Input: part model. Units: mm. Frame: model coordinates. Face numbers are marked on the shaded views. A direction names the side the tool comes from. Coordinates: 2 decimals unless noted, no trailing zeros. Loops run counter-clockwise (first coordinate to the right, second up) from the corner with the lowest first, then second, coordinate; pieces in that order, holes last. Notation, with made-up numbers: (-2, -23) -> (11, -23) arc R26 ccw to (11, -1) -> close; hole circle Ø4 at (56.25, -32). An arc over 180 degrees is marked (long way). Put each result on its own line as item: value. Start each with the question number.
1) Set-up query: the marked faces 1 and 2. Return all of +Z, -Z, +X, -X, +Y, -Y with unobstructed straight access to the full face (end or side cutting, diameter ignored); none if empty.
2) Cut plane A-A (x = 3.3). Return the cut outline in (y, z).
3) Cut plane D-D (y = 4.65). State how many separate pieces and enclosed holes the cut face has, plus the area to 3 significant figures.
4) Material intervals for L1, parallel to X at y = 3.35, z = -10; L2, parallel to X at y = 0.65, z = -8.5; L3, parallel to X at y = 1.15, z = -26, sorted ascending.
5) Cut plane B-B (x = 37). Return the cut outline in (y, z), plus the area to 3 significant figures.
6) Cut plane C-C (x = 56). Return the cut outline in (y, z), plus the area to 3 significant figures.
7) Contact query for flat-ended pins moving along their axis: P1, Ø1.5, axis at x = 26.5, y = 1.5, coming from the -Z side; P2, Ø3, axis at x = 16, z = -17.5, coming from the +Y side (3 decimals); P3, Ø3, axis at x = 25, z = -18.5, coming from the +Y side. Output: stop coordinate, or through.
from build123d import *

# Parameters (mm, degrees)
SKETCH_1_W                 = 60
SKETCH_1_H                 = 30
EXTRUDE_1_DEPTH            = 5.5
HOLE_WIZARD_41_D           = 2.9464
HOLE_WIZARD_41_CBORE_D     = 5.588
HOLE_WIZARD_41_CBORE_DEPTH = 2.9972
CUT_EXTRUDE_START          = -5.5
CUT_EXTRUDE_1_OUTLINE_R    = 2.25
CUT_EXTRUDE_1_OUTLINE_R_2  = 2
CUT_EXTRUDE_1_OUTLINE_R_3  = 1
CUT_EXTRUDE_1_DEPTH        = 5.5
CUT_EXTRUDE_START_2        = -3.5
SKETCH_4_3_R               = 5.5
SKETCH_4_3_R_2             = 2.25
CUT_EXTRUDE_2_DEPTH        = 3.5
CUT_EXTRUDE_START_3        = -3.3
CUT_EXTRUDE_3_DEPTH        = 3.3
HOLE_WIZARD_M3_AT_2_COUNT  = 2
HOLE_WIZARD_M3_AT_2_PITCH  = 14.637281168
HOLE_WIZARD_M3_AT_3_COUNT  = 2
HOLE_WIZARD_M3_AT_3_PITCH  = 36.045110625
HOLE_WIZARD_M3_AT_4_COUNT  = 2
HOLE_WIZARD_M3_AT_4_PITCH  = 33
SKETCH_7_R                 = 5
CUT_EXTRUDE_4_DEPTH        = 69.411439102


# Read off the part's stored shape, not the designer's step: the extrude step
with BuildPart() as part:
    # Sketch 1 → Extrude 1 (new body)
    with BuildSketch(Plane(origin=(0, 0, 0), x_dir=(1, 0, 0), z_dir=(0, 1, 0))):
        with Locations((30, 15)):
            Rectangle(SKETCH_1_W, SKETCH_1_H)
    extrude(amount=EXTRUDE_1_DEPTH)

    # Hole Wizard 41 (through all)
    with Locations(Plane(origin=(0, 5.5, 0), x_dir=(-1, 0, 0), z_dir=(0, 1, 0))):
        with Locations((-47.3, -9), (-3.3, -9), (-25.3, -18), (-3.3, -25), (-56.3, -9), (-56.3, -24)):
            CounterBoreHole(HOLE_WIZARD_41_D / 2, HOLE_WIZARD_41_CBORE_D / 2, HOLE_WIZARD_41_CBORE_DEPTH)

    # Cut-Extrude 1 outline → Cut-Extrude 1 (cut)
    with BuildSketch(Plane(origin=(0, 5.5, 0), x_dir=(1, 0, 0), z_dir=(0, 1, 0)).offset(CUT_EXTRUDE_START)):
        with BuildLine():
            Line((57.765087934, 30), (14.834912066, 30))
            ThreePointArc((14.834912066, 30), (36.3, 20.5), (57.765087934, 30))
        make_face()
        with Locations((36, 14.5)):
            Circle(CUT_EXTRUDE_1_OUTLINE_R)
        with Locations((19.3, 19.8)):
            Circle(CUT_EXTRUDE_1_OUTLINE_R_2)
        with Locations((33.1, 7.4)):
            Circle(CUT_EXTRUDE_1_OUTLINE_R_3)
        with Locations((38.9, 7.4)):
            Circle(CUT_EXTRUDE_1_OUTLINE_R_3)
        with Locations((56.3, 19.8)):
            Circle(CUT_EXTRUDE_1_OUTLINE_R_2)
    extrude(amount=CUT_EXTRUDE_1_DEPTH, mode=Mode.SUBTRACT)

    # Sketch 4_3 → Cut-Extrude 2 (cut)
    with BuildSketch(Plane(origin=(0, 5.5, 0), x_dir=(1, 0, 0), z_dir=(0, 1, 0)).offset(CUT_EXTRUDE_START_2)):
        with Locations(Location((36, 14.5, 0), (0, 0, 270))):
            Circle(SKETCH_4_3_R)
        with Locations(Location((36, 14.5, 0), (0, 0, 270))):
            Circle(SKETCH_4_3_R_2, mode=Mode.SUBTRACT)
    extrude(amount=CUT_EXTRUDE_2_DEPTH, mode=Mode.SUBTRACT)

    # Sketch 4_4 → Cut-Extrude 3 (cut)
    with BuildSketch(Plane(origin=(0, 5.5, 0), x_dir=(1, 0, 0), z_dir=(0, 1, 0)).offset(CUT_EXTRUDE_START_3)):
        with BuildLine():
            Line((39, 19.109772229), (39, 20.62596322))
            ThreePointArc((39, 20.62596322), (35.998381592, 20.501568554), (33, 20.688370404))
            Line((33, 20.688370404), (33, 19.109772229))
            ThreePointArc((33, 19.109772229), (36, 20), (39, 19.109772229))
        make_face()
    extrude(amount=CUT_EXTRUDE_3_DEPTH, mode=Mode.SUBTRACT)

    # Sketch 5 → Hole Wizard M3 (revolve, cut)
    with BuildSketch(Plane(origin=(18, 5.5, -3), x_dir=(0, 0, 1), z_dir=(1, 0, 0))):
        Polygon((0, 0), (0, 5.5), (1.525, 5.5), (1.25, 5.225), (1.25, 0.275), (1.525, 0), align=None)
    hole_wizard_m3 = revolve(axis=Axis((18, 11.85, -3), (0, -1, 0)), mode=Mode.SUBTRACT)

    # Hole Wizard M3 at 2: Hole Wizard M3 ×2
    with Locations(*[Vector(-0.1366373971370308, 0, -0.9906211292434749) * (i * HOLE_WIZARD_M3_AT_2_PITCH) for i in range(1, HOLE_WIZARD_M3_AT_2_COUNT)]):
        add(hole_wizard_m3, mode=Mode.SUBTRACT)

    # Hole Wizard M3 at 3: Hole Wizard M3 ×2
    with Locations(*[Vector(0.9155194540230326, 0, -0.40227369949496883) * (i * HOLE_WIZARD_M3_AT_3_PITCH) for i in range(1, HOLE_WIZARD_M3_AT_3_COUNT)]):
        add(hole_wizard_m3, mode=Mode.SUBTRACT)

    # Hole Wizard M3 at 4: Hole Wizard M3 ×2
    with Locations(*[(i * HOLE_WIZARD_M3_AT_4_PITCH, 0, 0) for i in range(1, HOLE_WIZARD_M3_AT_4_COUNT)]):
        add(hole_wizard_m3, mode=Mode.SUBTRACT)

    # Sketch 7 → Cut-Extrude 4 (cut, through all)
    with BuildSketch(Plane(origin=(0, 2.75, 2.75), x_dir=(-1, 0, 0), z_dir=(0, 0.7071067811865462, 0.7071067811865488))):
        with Locations(Location((-10.5, -9, 0), (0, 0, 90))):
            Circle(SKETCH_7_R)
    extrude(amount=-CUT_EXTRUDE_4_DEPTH, mode=Mode.SUBTRACT)


solid = part.part
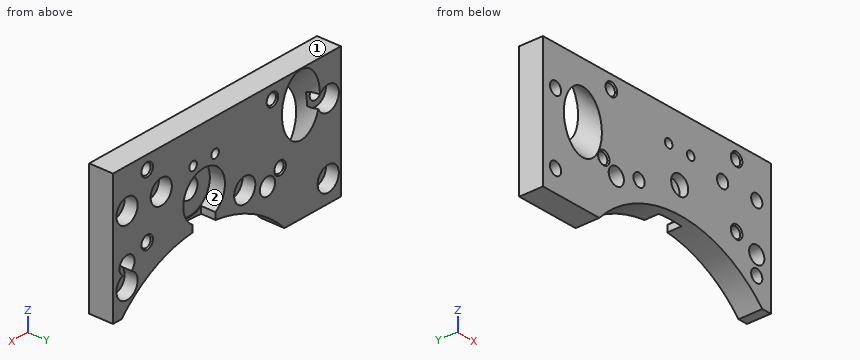
Results found:
1. face 1: +Z, +X, -X, +Y, -Y
1. face 2: +Y
2. outline: (0, -30) -> (5.5, -30) -> (5.5, -27.79) -> (2.5, -27.79) -> (2.5, -26.47) -> (0, -26.47) -> close; (0, -23.53) -> (2.5, -23.53) -> (2.5, -22.21) -> (5.5, -22.21) -> (5.5, -11.79) -> (2.5, -11.79) -> (2.5, -10.47) -> (0, -10.47) -> close; (0, -7.53) -> (2.5, -7.53) -> (2.5, -6.21) -> (5.5, -6.21) -> (5.5, 0) -> (0, 0) -> close
3. separate pieces: 1
3. enclosed holes: 13
3. area: 1,110 mm2
4. L1: x = 0 to 0.69, 15.48 to 32.84, 39.16 to 44.69, 49.91 to 53.69, 58.91 to 60
4. L2: x = 0 to 1.91, 4.69 to 6.19, 14.81 to 45.91, 48.69 to 54.91, 57.69 to 60
4. L3: x = 0 to 2.22, 4.38 to 19.31, 53.29 to 60
5. outline: (0, -20.51) -> (2.2, -20.51) -> (2.2, -19.91) -> (2, -19.91) -> (2, -16.52) -> (0, -16.52) -> close; (0, -12.48) -> (2, -12.48) -> (2, -9.09) -> (5.5, -9.09) -> (5.5, 0) -> (0, 0) -> close
5. area: 64.9 mm2
6. outline: (0, -28.22) -> (5.5, -28.22) -> (5.5, -26.78) -> (2.5, -26.78) -> (2.5, -25.44) -> (0, -25.44) -> close; (0, -22.56) -> (2.5, -22.56) -> (2.5, -21.78) -> (0, -21.78) -> close; (0, -17.82) -> (5.5, -17.82) -> (5.5, -11.78) -> (2.5, -11.78) -> (2.5, -10.44) -> (0, -10.44) -> close; (0, -7.56) -> (2.5, -7.56) -> (2.5, -6.22) -> (5.5, -6.22) -> (5.5, 0) -> (0, 0) -> close
6. area: 87.4 mm2
7. P1: stops at z = -22.49
7. P2: stops at y = 5.475
7. P3: stops at y = 2.5
